Job drawing, mm, ordinate dimensions from the low corner. One solid piece. Round coordinates to 2 decimals unless told otherwise and drop trailing zeros. Write each loop counter-clockwise with the first axis right and the second up, starting at its lowest first coordinate (ties: lowest second). Pieces come first, ordered by that corner, then holes.
1) Flat gauge pins, fed straight in: pin 1 (3 mm diameter, centred on x = 5.5, z = 7, fed in from -Y); pin 2 (2 mm diameter, centred on x = 28, y = 11.5, fed in from -Z); pin 3 (3 mm diameter, centred on y = 12, z = 10, fed in from -X); pin 4 (2 mm diameter, centred on y = 6, z = 3, fed in from +X). Where does each tip first touch, or does it go through?
2) Saw through at B-B (y = 24). Write the cut outline in (x, z), plus the area to 3 significant figures.
3) Pull direction X, two halves, no side cores. Call the marked faces 1, 2, 3 and 4: +X half, -X half, draft (parallel to the pull), parting line (faces both ways), or undercut.
4) Saw through at D-D (x = 33). Write the cut outline in (y, z), plus the area to 3 significant figures.
5) Wall check: probe 1 along Y at (x, z) = (19.05, 6.5) (3 decimals); probe 2 along X at (y, z) = (24, 11.5); probe 3 along X at (y, z) = (16.5, 1.5). Give the ranges that are in metal, low to high.
6) Saw through at A-A (x = 19.05). Write the cut outline in (y, z) (3 decimals), plus the area to 3 significant figures.
7) Saw through at C-C (z = 7.75). Write the cut outline in (x, y) (3 decimals).
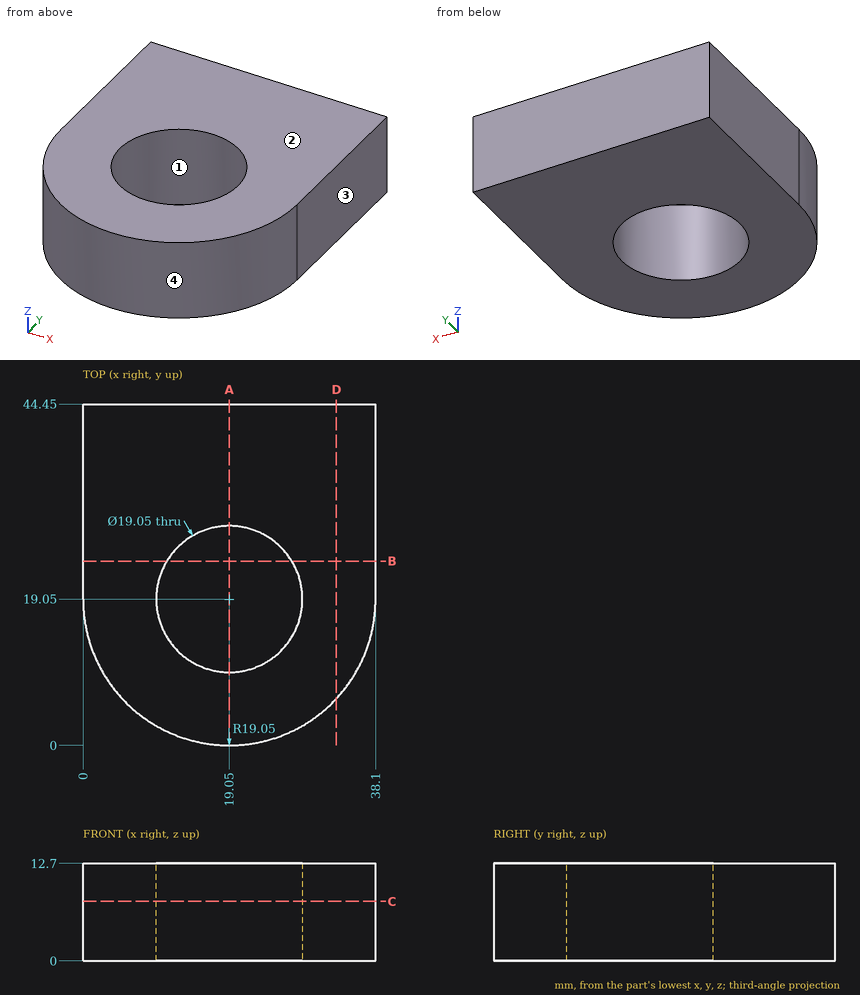
Evaluation:
1. pin 1: stops at y = 4.3
1. pin 2: stops at z = 0
1. pin 3: stops at x = 0.83
1. pin 4: stops at x = 33.8
2. outline: (0, 0) - (10.91, 0) - (10.91, 12.7) - (0, 12.7) - close; (27.19, 0) - (38.1, 0) - (38.1, 12.7) - (27.19, 12.7) - close
2. area: 277 mm2
3. face 1: undercut
3. face 2: draft
3. face 3: +X half
3. face 4: parting line
4. outline: (6.08, 0) - (44.45, 0) - (44.45, 12.7) - (6.08, 12.7) - close
4. area: 487 mm2
5. probe 1: y = 0 to 9.525, 28.575 to 44.45
5. probe 2: x = 0 to 10.91, 27.19 to 38.1
5. probe 3: x = 0.17 to 9.87, 28.23 to 37.93
6. outline: (0, 0) - (9.525, 0) - (9.525, 12.7) - (0, 12.7) - close; (28.575, 0) - (44.45, 0) - (44.45, 12.7) - (28.575, 12.7) - close
6. area: 323 mm2
7. outline: (0, 19.05) arc R19.05 ccw to (38.1, 19.05) - (38.1, 44.45) - (0, 44.45) - close; hole circle Ø19.05 at (19.05, 19.05)
